Source: CAD feature listing. Evaluate the final solid. Frame: model axes, mm. Face numbers are marked on the shaded views. A direction names the side the tool comes from. Round coordinates to 2 decimals unless told otherwise and drop trailing zeros. Write each loop counter-clockwise with the first axis right and the second up, starting at its lowest first coordinate (ties: lowest second). Pieces come first, ordered by that corner, then holes.
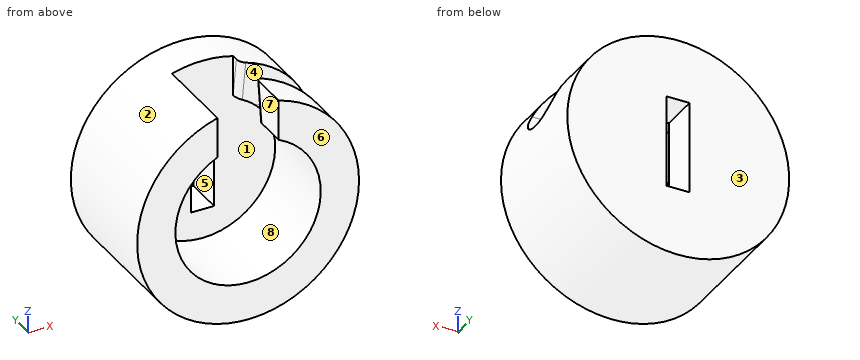
```python
from build123d import *

# Parameters (mm, degrees)
F0_R     = 7.25
F1_DEPTH = 8
F2_R     = 4.75
F3_DEPTH = 5.5
F4_W     = 4
F4_H     = 9.4417827204
F5_DEPTH = 5.5
F7_DEPTH = 7.251
F8_W     = 1.5
F8_H     = 6.0454548055
F9_DEPTH = 25
F10_R    = 0.4


with BuildPart() as f1:
    # F0 (on Front) → F1 (new body)
    with BuildSketch(Plane.XZ):
        Circle(F0_R)
    extrude(amount=F1_DEPTH)

    # F2 (on face) → F3 (cut)
    with BuildSketch(Plane.XZ.offset(8)):
        Circle(F2_R)
    extrude(amount=-F3_DEPTH, mode=Mode.SUBTRACT)

    # F4 (on face) → F5 (cut, through all)
    with BuildSketch(Plane.XZ.offset(8)):
        with BuildLine():
            Line((-2, 9.4417827204), (-2, 6.9686799324))
            ThreePointArc((-2, 6.9686799324), (0, 7.25), (2, 6.9686799324))
            Line((2, 6.9686799324), (2, 9.4417827204))
            Line((2, 9.4417827204), (-2, 9.4417827204))
        make_face()
        with Locations((0, 4.7208913602)):
            Rectangle(F4_W, F4_H)
    extrude(amount=-F5_DEPTH, mode=Mode.SUBTRACT)

    # F6 (on Right) → F7 (cut, through all)
    with BuildSketch(Plane.YZ):
        with BuildLine():
            Line((-5.0896294415, 7.9721454531), (-5.7264296338, 3.302275436))
            ThreePointArc((-5.7264296338, 3.302275436), (-4.1996874086, 1.6687326956), (-2.7646700478, 3.3834130977))
            Line((-2.7646700478, 3.3834130977), (-3.4622503445, 8.0075236037))
            Line((-3.4622503445, 8.0075236037), (-5.0896294415, 7.9721454531))
        make_face()
    extrude(amount=F7_DEPTH, mode=Mode.SUBTRACT)

    # F8 (on face) → F9 (cut)
    with BuildSketch(Plane.XZ):
        with Locations((0.0068399386, 0.2177511924)):
            Rectangle(F8_W, F8_H)
    extrude(amount=F9_DEPTH, mode=Mode.SUBTRACT)

    # F10
    f10_edges = [f1.edges().sort_by_distance(p)[0] for p in [
        (2, -3.104874, 5.638551),
        (2, -5.407847, 5.638551),
    ]]
    fillet(f10_edges, radius=F10_R)


solid = f1.part
```
Q1. Pin query (flat end, axial travel): P1, Ø0.7, axis at y = -6.5, z = 5, coming from the -X side; P2, Ø2, axis at x = -0.5, z = 2, coming from the -Y side; P3, Ø1.8, axis at y = -4.24, z = 3.16, coming from the +X side. Return the tip coordinate at first contact, or that it passes through.
Q2. Section query D-D, the plane z = 2.5. Output: boundary loops of the cut face in (x, y), and give its area (3 significant figures).
Q3. Line query: line 1 (X direction, y = -5.5, z = 0); line 2 (Y direction, x = -2.5, z = -3.5); line 3 (Y direction, x = 3.75, z = 3). Output: solid intervals per line, ascending.
Q4. Section query A-A, the plane z = 0. Output: boundary loops of the cut face in (x, y).
Q5. Set-up query: the marked faces 4, 5, 6, 7 and 8. Return all of +Z, -Z, +X, -X, +Y, -Y with unobstructed straight access to the full face (end or side cutting, diameter ignored); none if empty.
Q6. Section query C-C, the plane y = -1.5. Output: boundary loops of the cut face in (x, z), and give its area (3 significant figures).
Q7. Mould query, pull axis Z, two halves, no side actions, for the marked faces 1, 2 and 3. Classes: pulls with the +Z half, pulls with the -Z half, needs draft (parallel to the pull), parting line crosses it, or undercut.
Q8. Section query B-B, the plane x = 0. Output: boundary loops of the cut face in (y, z), and give its area (3 significant figures).
Filled in:
1. P1: stops at x = -5.56
1. P2: stops at y = -2.5
1. P3: stops at x = -2.47
2. outline: (-6.81, -8) - (-4.04, -8) - (-4.04, -2.5) - (-0.74, -2.5) - (-0.74, 0) - (-6.81, 0) - close; (0.76, -2.5) - (4.04, -2.5) - (4.04, -2.9) - (6.81, -2.9) - (6.81, 0) - (0.76, 0) - close; (4.04, -8) - (6.81, -8) - (6.81, -5.58) - (4.04, -5.58) - close
2. area: 53.3 mm2
3. line 1: x = -7.25 to -4.75, 4.75 to 7.25
3. line 2: y = -2.5 to 0
3. line 3: y = -8 to -5.72, -2.76 to 0
4. outline: (-7.25, -8) - (-4.75, -8) - (-4.75, -2.5) - (-0.74, -2.5) - (-0.74, 0) - (-7.25, 0) - close; (0.76, -2.5) - (4.75, -2.5) - (4.75, -8) - (7.25, -8) - (7.25, 0) - (0.76, 0) - close
5. face 4: +X
5. face 5: +Y, -Y
5. face 6: +Z, -Z, +X, -X, -Y
5. face 7: +Z, -Y
5. face 8: -Y
6. outline: circle Ø14.5 at (0, 0); hole (-0.74, -2.8) - (0.76, -2.8) - (0.76, 3.24) - (-0.74, 3.24) - close
6. area: 156 mm2
7. face 1: undercut
7. face 2: parting line crosses it
7. face 3: needs draft
8. outline: (-8, -7.25) - (0, -7.25) - (0, -2.8) - (-2.5, -2.8) - (-2.5, -4.75) - (-8, -4.75) - close; (-2.5, 3.24) - (0, 3.24) - (0, 7.25) - (-2.5, 7.25) - close
8. area: 34.9 mm2
